Source: CAD feature listing. Evaluate the final solid. Frame: model axes, mm. A direction names the side the tool comes from. Round coordinates to 2 decimals unless told otherwise and drop trailing zeros. Write each question's results on one line, items separated by ' | '. Start each with the question number.
1. Set-up query: faces 3 (the flat face through (-20, -10, 126)), 4 (the flat face through (-8.6, -7.1, 125.7)), 5 (the flat face through (0, -5.5, 126)). Return all of +Z, -Z, +X, -X, +Y, -Y with unobstructed straight access to the full face (end or side cutting, diameter ignored); none if empty.
2. Section A-A on z = 167. Give the number of separate pieces and of enclosed holes in the cut face, and give its area (3 significant figures).
3. Contact query for flat-ended pins moving along their axis: pin 1 Ø0.8 at (y, z) = (-17, 5.5) entering from +X; pin 2 Ø5 at (y, z) = (2, 212) entering from -X; pin 3 Ø0.8 at (y, z) = (-19.5, 82) entering from +X. Output: stop coordinate, or through.
4. Ray query, line 1 (Y direction, x = 16, z = 46); line 2 (Y direction, x = 15, z = 128). Return the intervals inside material, ascending.
5. Draft query along Z for faces 1 (the cylindrical face through (11.15, 14.39, 12.22)), 2 (the flat face through (-10.19, -15, 4)). Return one class per face: released by +Z, released by -Z, zero draft, split by the parting line, or undercut.
from build123d import *

# Parameters (mm, degrees)
BOSS_EXTRUDE1_DEPTH     = 255
MIRROR3_COPY_1_DEPTH    = 255
MIRROR3_COPY_2_DEPTH    = 255
SKETCH2_R               = 2.5
CUT_EXTRUDE1_DEPTH      = 15.5
CUT_EXTRUDE1_DEPTH_BACK = 26.5


with BuildPart() as part:
    # Sketch1 → Boss-Extrude1 (new body)
    with BuildSketch(Plane.XY):
        with BuildLine():
            Line((3.4, 0), (5.5, 0))
            Line((5.5, 0), (5.5, 4))
            Line((5.5, 4), (11.69, 10.19))
            Line((11.69, 10.19), (18.2, 10.19))
            Line((18.2, 10.19), (18.2, 5.265595036))
            Line((18.2, 5.265595036), (15.5, 5.265595036))
            Line((15.5, 5.265595036), (15.5, 2.965595036))
            Line((15.5, 2.965595036), (19, 2.965595036))
            Line((19, 2.965595036), (19, 3.965595036))
            Line((19, 3.965595036), (20, 3.965595036))
            Line((20, 3.965595036), (20, 15.5))
            ThreePointArc((20, 15.5), (18.681980515, 18.681980515), (15.5, 20))
            Line((15.5, 20), (6.385304712, 20))
            Line((6.385304712, 20), (6.385304712, 19))
            Line((6.385304712, 19), (5.385304712, 19))
            Line((5.385304712, 19), (5.385304712, 15.5))
            Line((5.385304712, 15.5), (7.685304712, 15.5))
            Line((7.685304712, 15.5), (7.685304712, 18.2))
            Line((7.685304712, 18.2), (10.19, 18.2))
            Line((10.19, 18.2), (10.19, 11.69))
            Line((10.19, 11.69), (4, 5.5))
            Line((4, 5.5), (0, 5.5))
            Line((0, 5.5), (0, 3.4))
            ThreePointArc((0, 3.4), (2.404163056, 2.404163056), (3.4, 0))
        make_face()
        with BuildLine():
            Line((18.5, 11.69), (18.5, 15.5))
            ThreePointArc((18.5, 15.5), (17.621320344, 17.621320344), (15.5, 18.5))
            Line((15.5, 18.5), (11.69, 18.5))
            Line((11.69, 18.5), (11.69, 11.69))
            Line((11.69, 11.69), (18.5, 11.69))
        make_face(mode=Mode.SUBTRACT)
    boss_extrude1 = extrude(amount=BOSS_EXTRUDE1_DEPTH)

    # Mirror1: Boss-Extrude1 across plane
    add(boss_extrude1.mirror(Plane.ZX))

    # Mirror2: Boss-Extrude1 across plane
    add(boss_extrude1.mirror(Plane(origin=(0, 0, 0), x_dir=(0, 0, 1), z_dir=(1, 0, 0))))

    # Mirror3 copy 1 sketch → Mirror3 copy 1 (add)
    with BuildSketch(Plane(origin=(0, 0, 0), x_dir=(-1, 0, 0), z_dir=(0, 0, 1))):
        with BuildLine():
            Line((3.4, 0), (5.5, 0))
            Line((5.5, 0), (5.5, 4))
            Line((5.5, 4), (11.69, 10.19))
            Line((11.69, 10.19), (18.2, 10.19))
            Line((18.2, 10.19), (18.2, 5.265595036))
            Line((18.2, 5.265595036), (15.5, 5.265595036))
            Line((15.5, 5.265595036), (15.5, 2.965595036))
            Line((15.5, 2.965595036), (19, 2.965595036))
            Line((19, 2.965595036), (19, 3.965595036))
            Line((19, 3.965595036), (20, 3.965595036))
            Line((20, 3.965595036), (20, 15.5))
            ThreePointArc((20, 15.5), (18.681980515, 18.681980515), (15.5, 20))
            Line((15.5, 20), (6.385304712, 20))
            Line((6.385304712, 20), (6.385304712, 19))
            Line((6.385304712, 19), (5.385304712, 19))
            Line((5.385304712, 19), (5.385304712, 15.5))
            Line((5.385304712, 15.5), (7.685304712, 15.5))
            Line((7.685304712, 15.5), (7.685304712, 18.2))
            Line((7.685304712, 18.2), (10.19, 18.2))
            Line((10.19, 18.2), (10.19, 11.69))
            Line((10.19, 11.69), (4, 5.5))
            Line((4, 5.5), (0, 5.5))
            Line((0, 5.5), (0, 3.4))
            ThreePointArc((0, 3.4), (2.404163056, 2.404163056), (3.4, 0))
        make_face()
        with BuildLine():
            Line((18.5, 11.69), (18.5, 15.5))
            ThreePointArc((18.5, 15.5), (17.621320344, 17.621320344), (15.5, 18.5))
            Line((15.5, 18.5), (11.69, 18.5))
            Line((11.69, 18.5), (11.69, 11.69))
            Line((11.69, 11.69), (18.5, 11.69))
        make_face(mode=Mode.SUBTRACT)
    extrude(amount=MIRROR3_COPY_1_DEPTH)

    # Mirror3 copy 2 sketch → Mirror3 copy 2 (add)
    with BuildSketch(Plane.XY):
        with BuildLine():
            Line((3.4, 0), (5.5, 0))
            Line((5.5, 0), (5.5, -4))
            Line((5.5, -4), (11.69, -10.19))
            Line((11.69, -10.19), (18.2, -10.19))
            Line((18.2, -10.19), (18.2, -5.265595036))
            Line((18.2, -5.265595036), (15.5, -5.265595036))
            Line((15.5, -5.265595036), (15.5, -2.965595036))
            Line((15.5, -2.965595036), (19, -2.965595036))
            Line((19, -2.965595036), (19, -3.965595036))
            Line((19, -3.965595036), (20, -3.965595036))
            Line((20, -3.965595036), (20, -15.5))
            ThreePointArc((20, -15.5), (18.681980515, -18.681980515), (15.5, -20))
            Line((15.5, -20), (6.385304712, -20))
            Line((6.385304712, -20), (6.385304712, -19))
            Line((6.385304712, -19), (5.385304712, -19))
            Line((5.385304712, -19), (5.385304712, -15.5))
            Line((5.385304712, -15.5), (7.685304712, -15.5))
            Line((7.685304712, -15.5), (7.685304712, -18.2))
            Line((7.685304712, -18.2), (10.19, -18.2))
            Line((10.19, -18.2), (10.19, -11.69))
            Line((10.19, -11.69), (4, -5.5))
            Line((4, -5.5), (0, -5.5))
            Line((0, -5.5), (0, -3.4))
            ThreePointArc((0, -3.4), (2.404163056, -2.404163056), (3.4, 0))
        make_face()
        with BuildLine():
            Line((18.5, -11.69), (18.5, -15.5))
            ThreePointArc((18.5, -15.5), (17.621320344, -17.621320344), (15.5, -18.5))
            Line((15.5, -18.5), (11.69, -18.5))
            Line((11.69, -18.5), (11.69, -11.69))
            Line((11.69, -11.69), (18.5, -11.69))
        make_face(mode=Mode.SUBTRACT)
    extrude(amount=MIRROR3_COPY_2_DEPTH)

    # Sketch2 → Cut-Extrude1 (cut, two sides)
    with BuildSketch(Plane(origin=(0, 5.5, 0), x_dir=(1, 0, 0), z_dir=(0, 1, 0))) as cut_extrude1_sk:
        with Locations((-10, -10)):
            Circle(SKETCH2_R)
        with Locations((10, -10)):
            Circle(SKETCH2_R)
    extrude(amount=CUT_EXTRUDE1_DEPTH, mode=Mode.SUBTRACT)
    extrude(cut_extrude1_sk.sketch, amount=-CUT_EXTRUDE1_DEPTH_BACK, mode=Mode.SUBTRACT)


solid = part.part
Taken from the geometry:
1) face 3: +Z, -Z, -X, +Y, -Y | face 4: +Z, -Z | face 5: +Z, -Z, -Y
2) separate pieces: 1 | enclosed holes: 5 | area: 468 mm^2
3) pin 1: x = 19.86 | pin 2: x = -20 | pin 3: x = 18.2
4) line 1: -19.97 to -18.46, -11.69 to -10.19, -5.27 to -2.97, 2.97 to 5.27, 10.19 to 11.69, 18.46 to 19.97 | line 2: -20 to -18.5, -11.69 to -10.19, 10.19 to 11.69, 18.5 to 20
5) face 1: undercut | face 2: zero draft
